Geometry check sheet. Reference: the model listing, model coordinates, mm. A direction names the side the tool comes from. Give positions to 0.01 mm unless a question says otherwise; leave off trailing zeros. Loops run counter-clockwise (first coordinate to the right, second up) from the corner with the lowest first, then second, coordinate; pieces in that order, holes last. Notation, with made-up numbers: (26.5, 24) - (76.5, 24) arc R28 cw to (76.5, 56) - close; hole circle Ø2 at (-23.75, -19). An arc over 180 degrees is marked (long way). Write item = value, one per line. Start each with the question number.
from build123d import *

# Parameters (mm, degrees)
SALIENTE_EXTRUIR3_DEPTH      = 27.5
SALIENTE_EXTRUIR4_REACH      = 167.17
SALIENTE_EXTRUIR4_END_RADIUS = 50
CROQUIS2_R                   = 25
CROQUIS5_R                   = 45
CROQUIS5_R_2                 = 32.5
CORTAR_EXTRUIR2_DEPTH        = 2.5
CROQUIS6_R                   = 10.5
CORTAR_EXTRUIR3_DEPTH        = 172.901134438
CORTAR_EXTRUIR4_DEPTH        = 20
CROQUIS8_R                   = 30
CORTAR_EXTRUIR5_DEPTH        = 27
CROQUIS9_R                   = 1.5
CORTAR_EXTRUIR7_DEPTH        = 30
CROQUIS10_R                  = 12.5
CORTAR_EXTRUIR8_DEPTH        = 5
CROQUIS11_R                  = 1.5
CORTAR_EXTRUIR9_DEPTH        = 172.117649646
CORTAR_EXTRUIR10_DEPTH       = 20
CROQUIS13_R                  = 1.5
CORTAR_EXTRUIR11_DEPTH       = 167.583312541
CROQUIS14_R                  = 17.5
CROQUIS14_R_2                = 10
CORTAR_EXTRUIR12_DEPTH       = 2
CROQUIS15_R                  = 13.5
CROQUIS15_R_2                = 10
CORTAR_EXTRUIR13_DEPTH       = 4


with BuildPart() as part:
    # Croquis3 → Saliente-Extruir3 (new, symmetric)
    with BuildSketch(Plane(origin=(0, 0, 0), x_dir=(0, 0, -1), z_dir=(1, 0, 0))):
        with BuildLine():
            Line((-50, 105), (-50, 70))
            ThreePointArc((-50, 70), (0, 20), (50, 70))
            Line((50, 70), (50, 105))
            ThreePointArc((50, 105), (0, 155), (-50, 105))
        make_face()
    extrude(amount=SALIENTE_EXTRUIR3_DEPTH, both=True)

    # Saliente-Extruir4: up to this cylinder (the profile starts outside it)
    saliente_extruir4_end = Plane(origin=(0, 70, 0), z_dir=(-1, 0, 0)) * Cylinder(SALIENTE_EXTRUIR4_END_RADIUS, 435.34, mode=Mode.PRIVATE)
    # Croquis2 → Saliente-Extruir4 (add, up to the surface)
    with BuildSketch(Plane(origin=(0, 0, 0), x_dir=(1, 0, 0), z_dir=(0, 1, 0)), mode=Mode.PRIVATE) as saliente_extruir4_sk1:
        with Locations(Location((0, 0, 0), (0, 0, 90))):
            Circle(CROQUIS2_R)
    saliente_extruir4_tool1 = extrude(saliente_extruir4_sk1.sketch, amount=SALIENTE_EXTRUIR4_REACH, mode=Mode.PRIVATE) - saliente_extruir4_end
    add(saliente_extruir4_tool1.solids().sort_by_distance((0, 0, 0))[0])

    # Croquis5 → Cortar-Extruir2 (cut)
    with BuildSketch(Plane.ZY.offset(27.5)):
        with Locations((0, 105)):
            Circle(CROQUIS5_R)
        with Locations((0, 105)):
            Circle(CROQUIS5_R_2, mode=Mode.SUBTRACT)
    extrude(amount=-CORTAR_EXTRUIR2_DEPTH, mode=Mode.SUBTRACT)

    # Croquis6 → Cortar-Extruir3 (cut, through all)
    with BuildSketch(Plane.ZY.offset(27.5)):
        with Locations((0, 105)):
            Circle(CROQUIS6_R)
    extrude(amount=-CORTAR_EXTRUIR3_DEPTH, mode=Mode.SUBTRACT)

    # Croquis7 → Cortar-Extruir4 (cut)
    with BuildSketch(Plane(origin=(27.5, 0, 0), x_dir=(0, 0, -1), z_dir=(1, 0, 0))):
        with BuildLine():
            Line((-50, 105), (-50, 70))
            ThreePointArc((-50, 70), (0, 20), (50, 70))
            Line((50, 70), (50, 105))
            ThreePointArc((50, 105), (0, 155), (-50, 105))
        make_face()
    extrude(amount=-CORTAR_EXTRUIR4_DEPTH, mode=Mode.SUBTRACT)

    # Croquis8 → Cortar-Extruir5 (cut)
    with BuildSketch(Plane(origin=(7.5, 0, 0), x_dir=(0, 0, -1), z_dir=(1, 0, 0))):
        with Locations((0, 105)):
            Circle(CROQUIS8_R)
    extrude(amount=-CORTAR_EXTRUIR5_DEPTH, mode=Mode.SUBTRACT)

    # Croquis9 → Cortar-Extruir7 (cut)
    with BuildSketch(Plane.XZ):
        with Locations(Location((7.5, 0, 0), (0, 0, 270))):
            Circle(CROQUIS9_R)
        with Locations(Location((3.75, -6.495190528, 0), (0, 0, 270))):
            Circle(CROQUIS9_R)
        with Locations(Location((-3.75, -6.495190528, 0), (0, 0, 270))):
            Circle(CROQUIS9_R)
        with Locations(Location((-7.5, 0, 0), (0, 0, 270))):
            Circle(CROQUIS9_R)
        with Locations(Location((-3.75, 6.495190528, 0), (0, 0, 270))):
            Circle(CROQUIS9_R)
        with Locations(Location((3.75, 6.495190528, 0), (0, 0, 270))):
            Circle(CROQUIS9_R)
    extrude(amount=-CORTAR_EXTRUIR7_DEPTH, mode=Mode.SUBTRACT)

    # Croquis10 → Cortar-Extruir8 (cut)
    with BuildSketch(Plane(origin=(0, 26, 0), x_dir=(1, 0, 0), z_dir=(0, 1, 0))):
        Circle(CROQUIS10_R)
    extrude(amount=CORTAR_EXTRUIR8_DEPTH, mode=Mode.SUBTRACT)

    # Croquis11 → Cortar-Extruir9 (cut, through all)
    with BuildSketch(Plane.ZY.offset(27.5)):
        with Locations((27.5, 105)):
            Circle(CROQUIS11_R)
        with Locations((17.145969551, 83.499634232)):
            Circle(CROQUIS11_R)
        with Locations((-6.119325684, 78.189482415)):
            Circle(CROQUIS11_R)
        with Locations((-24.776643867, 93.068197174)):
            Circle(CROQUIS11_R)
        with Locations((-24.776643867, 116.931802826)):
            Circle(CROQUIS11_R)
        with Locations((-6.119325684, 131.810517585)):
            Circle(CROQUIS11_R)
        with Locations((17.145969551, 126.500365768)):
            Circle(CROQUIS11_R)
    extrude(amount=-CORTAR_EXTRUIR9_DEPTH, mode=Mode.SUBTRACT)

    # Croquis12 → Cortar-Extruir10 (cut)
    with BuildSketch(Plane(origin=(7.5, 0, 0), x_dir=(0, 0, -1), z_dir=(1, 0, 0))):
        with BuildLine():
            ThreePointArc((-34.641016151, 85), (0, 25), (34.641016151, 85))
            ThreePointArc((34.641016151, 85), (0, 65), (-34.641016151, 85))
        make_face()
    extrude(amount=-CORTAR_EXTRUIR10_DEPTH, mode=Mode.SUBTRACT)

    # Croquis13 → Cortar-Extruir11 (cut, through all)
    with BuildSketch(Plane(origin=(7.5, 0, 0), x_dir=(0, 0, -1), z_dir=(1, 0, 0))):
        with Locations((0, 152.5)):
            Circle(CROQUIS13_R)
        with Locations((47.5, 105)):
            Circle(CROQUIS13_R)
        with Locations((-47.5, 105)):
            Circle(CROQUIS13_R)
        with Locations((-47.5, 70)):
            Circle(CROQUIS13_R)
        with Locations((47.5, 70)):
            Circle(CROQUIS13_R)
        with Locations((33.587572106, 36.412427894)):
            Circle(CROQUIS13_R)
        with Locations((-33.587572106, 36.412427894)):
            Circle(CROQUIS13_R)
    extrude(amount=-CORTAR_EXTRUIR11_DEPTH, mode=Mode.SUBTRACT)

    # Croquis14 → Cortar-Extruir12 (cut)
    with BuildSketch(Plane.XZ):
        with Locations(Location((0, 0, 0), (0, 0, 270))):
            Circle(CROQUIS14_R)
        with Locations(Location((0, 0, 0), (0, 0, 270))):
            Circle(CROQUIS14_R_2, mode=Mode.SUBTRACT)
    extrude(amount=-CORTAR_EXTRUIR12_DEPTH, mode=Mode.SUBTRACT)

    # Croquis15 → Cortar-Extruir13 (cut)
    with BuildSketch(Plane.ZY.offset(27.5)):
        with Locations((0, 105)):
            Circle(CROQUIS15_R)
        with Locations((0, 105)):
            Circle(CROQUIS15_R_2, mode=Mode.SUBTRACT)
    extrude(amount=-CORTAR_EXTRUIR13_DEPTH, mode=Mode.SUBTRACT)


solid = part.part
1) Release check for a two-part mould opening along Y. For faces 6 (the face through (-10, 88, 50)), 7 (the face through (-17.533, 23.403, 18.13)), 8 (the face through (-2.36, 65.004, -0.586)) record: pulls with the +Y half, pulls with the -Y half, needs draft (parallel to the pull), parting line crosses it, or undercut.
2) Gauge pin test, flat ends, axial feed: P1, Ø4, axis at y = 105, z = 47.5, coming from the +X side; P2, Ø6, axis at y = 25.5, z = -19.5, coming from the +X side; P3, Ø10, axis at x = -11.5, z = 18.5, coming from the +Y side; P4, Ø1.5, axis at x = -1.5, z = 4.5, coming from the -Y side. Record the tip position at first contact, or that the pin passes through.
3) Cross-section at B-B on y = 87.5. Enter the section's corners in (x, z), and give its area (3 significant figures).
4) Material ranges on line 1 along Y through (x, z) = (3.25, 0); line 2 along Y through (x, z) = (-14.5, 0); line 3 along Z through (x, y) = (-9, 70), recorded low to high.
5) Cross-section at A-A on x = -21.5. Give the number of separate pieces and of enclosed holes in the cut face, and give its area (3 significant figures).
6) Cross-section at D-D on y = 142.5. Enter the section's corners in (x, z), and give its area (3 significant figures).
7) Cross-section at C-C on x = 14. Enter the section's corners in (y, z), and give its area (3 significant figures).
8) Tool access check on faces 1 (the face through (5, 0, 17)), 2 (the face through (-7.509, 10.196, -23.846)), 3 (the face through (-0.98, 26.38, 12.46)), 4 (the face through (-25.53, 116.38, 7.26)), 5 (the face through (-10, 70, 49)). Record the directions out of +Z, -Z, +X, -X, +Y, -Y that give a thin tool (end or side, any length) a straight path to the whole face; none if there is none.
Checked values:
q1.face_6 = needs draft
q1.face_7 = pulls with the -Y half
q1.face_8 = undercut
q2.P1 = 7.5
q2.P2 = 17.77
q2.P3 = 153.14
q2.P4 = 0
q3.outline = (-27.5, -50) - (7.5, -50) - (7.5, -24.37) - (-19.5, -24.37) - (-19.5, 24.37) - (7.5, 24.37) - (7.5, 50) - (-27.5, 50) - (-27.5, 41.46) - (-25, 41.46) - (-25, 27.39) - (-27.5, 27.39) - (-27.5, -27.39) - (-25, -27.39) - (-25, -41.46) - (-27.5, -41.46) - close
q3.area = 2,110 mm²
q4.line_1 = 0 to 25, 65 to 75, 135 to 151, 154 to 155
q4.line_2 = 2 to 75, 135 to 151, 154 to 155
q4.line_3 = -50 to -49, -46 to -39.69, -19.36 to 19.36, 39.69 to 46, 49 to 50
q5.separate_pieces = 1
q5.enclosed_holes = 15
q5.area = 11,400 mm²
q6.outline = (-27.5, -33.07) - (7.5, -33.07) - (7.5, 33.07) - (-27.5, 33.07) - (-27.5, 24.87) - (-25, 24.87) - (-25, -24.87) - (-27.5, -24.87) - close
q6.area = 2,190 mm²
q7.outline = (0, -20.71) - (24.49, -20.71) arc R50 cw to (24.49, 20.71) - (0, 20.71) - (0, 10.5) - (2, 10.5) - (2, -10.5) - (0, -10.5) - close
q7.area = 847 mm²
q8.face_1 = +Z, -Z, +X, -X, -Y
q8.face_2 = -Y
q8.face_3 = none
q8.face_4 = -X
q8.face_5 = +X, -X
